The listing builds one solid part. Answer for the finished solid, in the listing's coordinates (mm). A direction names the side the tool comes from. Give positions to 0.01 mm unless a question says otherwise; leave off trailing zeros. Order: outer loops, then holes, each group sorted by start corner. A loop starts at its lowest first (then second) coordinate and runs counter-clockwise, first axis right, second up. Notation, with made-up numbers: (74, -13.5) -> (119, -13.5) arc R11 ccw to (119, -7.5) -> close; hole circle Ø8 at (87.5, 64.5). An arc over 180 degrees is marked (long way). Write item = value, one per line. Start each with the question number.
```python
from build123d import *

# Parameters (mm, degrees)
F1_DEPTH = 45
F0_R     = 1.2
F2_DEPTH = 1.5


with BuildPart() as f1:
    # F0 (on Top) → F1 (new body)
    with BuildSketch(Plane.XY):
        with BuildLine():
            Line((-13.376313, -16.508007), (-13.376313, -5.371486))
            ThreePointArc((-13.376313, -5.371486), (-27.376313, -1.436818), (-41.376313, -5.371486))
            Line((-41.376313, -5.371486), (-41.376313, -16.508007))
            ThreePointArc((-41.376313, -16.508007), (-27.376313, -20.442675), (-13.376313, -16.508007))
        make_face()
        with BuildLine():
            Line((-40.376313, -15.939747), (-40.376313, -5.939747))
            ThreePointArc((-40.376313, -5.939747), (-27.376313, -2.436818), (-14.376313, -5.939747))
            Line((-14.376313, -5.939747), (-14.376313, -15.939747))
            ThreePointArc((-14.376313, -15.939747), (-27.376313, -19.442675), (-40.376313, -15.939747))
        make_face(mode=Mode.SUBTRACT)
    extrude(amount=F1_DEPTH)

    # F0 (on Top) → F2 (join)
    with BuildSketch(Plane.XY):
        with BuildLine():
            ThreePointArc((-14.376313, -5.939747), (-27.376313, -2.436818), (-40.376313, -5.939747))
            Line((-40.376313, -5.939747), (-40.376313, -15.939747))
            ThreePointArc((-40.376313, -15.939747), (-27.376313, -19.442675), (-14.376313, -15.939747))
            Line((-14.376313, -15.939747), (-14.376313, -5.939747))
        make_face()
        with Locations((-32.828095, -16.290346)):
            Circle(F0_R, mode=Mode.SUBTRACT)
        with Locations((-28.928095, -16.290346)):
            Circle(F0_R, mode=Mode.SUBTRACT)
        with Locations((-36.702558, -12.947978)):
            Circle(F0_R, mode=Mode.SUBTRACT)
        with Locations((-32.828095, -12.947978)):
            Circle(F0_R, mode=Mode.SUBTRACT)
        with Locations((-28.928095, -12.947978)):
            Circle(F0_R, mode=Mode.SUBTRACT)
        with Locations((-25.028095, -16.290346)):
            Circle(F0_R, mode=Mode.SUBTRACT)
        with Locations((-21.128095, -16.290346)):
            Circle(F0_R, mode=Mode.SUBTRACT)
        with Locations((-25.028095, -12.947978)):
            Circle(F0_R, mode=Mode.SUBTRACT)
        with Locations((-21.128095, -12.947978)):
            Circle(F0_R, mode=Mode.SUBTRACT)
        with Locations((-17.228095, -12.947978)):
            Circle(F0_R, mode=Mode.SUBTRACT)
        with Locations((-36.702558, -9.047978)):
            Circle(F0_R, mode=Mode.SUBTRACT)
        with Locations((-32.828095, -9.047978)):
            Circle(F0_R, mode=Mode.SUBTRACT)
        with Locations((-28.928095, -9.047978)):
            Circle(F0_R, mode=Mode.SUBTRACT)
        with Locations((-32.828095, -5.190346)):
            Circle(F0_R, mode=Mode.SUBTRACT)
        with Locations((-28.928095, -5.190346)):
            Circle(F0_R, mode=Mode.SUBTRACT)
        with Locations((-25.028095, -9.047978)):
            Circle(F0_R, mode=Mode.SUBTRACT)
        with Locations((-21.128095, -9.047978)):
            Circle(F0_R, mode=Mode.SUBTRACT)
        with Locations((-17.228095, -9.047978)):
            Circle(F0_R, mode=Mode.SUBTRACT)
        with Locations((-25.028095, -5.190346)):
            Circle(F0_R, mode=Mode.SUBTRACT)
        with Locations((-21.128095, -5.190346)):
            Circle(F0_R, mode=Mode.SUBTRACT)
    extrude(amount=F2_DEPTH)


solid = f1.part
```
Item 1: A cutting plane is placed at B-B, the plane x = -32.25. Write down the section's boundary in (y, z).
Item 2: Consider L1, parallel to X at y = -13.75, z = 43; L2, parallel to Y at x = -28, z = 40; L3, parallel to Z at x = -37.5, y = -16.5. Determine where each line is inside the solid, lowest interval first. Write a range as from..to.
Item 3: A cutting plane is placed at C-C, the plane x = -36.5. Write down the section's boundary in (y, z), plus the area to 3 significant figures.
Item 4: The mould has two halves that part along X. Classify faces 3 (the flat face through (-41.376, -11, 22)), 4 (the cylindrical face through (-27.17, -1.438, 22.185)), 5 (the cylindrical face through (-16.084, -12.588, 0.74)): +X half, -X half, draft (parallel to the pull), parting line (faces both ways), or undercut.
Item 5: Which of the six approach directions +Z, -Z, +X, -X, +Y, -Y give full straight-line access (tool end or side, diameter ignored) to faces 1 (the cylindrical face through (-27.186, -19.442, 22.946)), 2 (the cylindrical face through (-22.327, -5.138, 0.74))?
Item 6: Flat-ended cylindrical pins translate along their axes: pin 1 (4 mm diameter, centred on x = -32.83, y = -12.95, fed in from +Z); pin 2 (4 mm diameter, centred on x = -31.5, z = 35.5, fed in from -Y); pin 3 (1.5 mm diameter, centred on x = -30.5, z = 10, fed in from -Y). Find the tip coordinate at first contact, or state that the pin passes through.
Item 7: A cutting plane is placed at A-A, the plane z = 19.5. Write down the section's boundary in (x, y), plus the area to 3 significant figures.
Item 8: A cutting plane is placed at D-D, the plane x = -28.5. Write down the section's boundary in (y, z), plus the area to 3 significant figures.
Check values:
q1.outline = (-20, 0) -> (-17.34, 0) -> (-17.34, 1.5) -> (-18.98, 1.5) -> (-18.98, 45) -> (-20, 45) -> close; (-15.24, 0) -> (-14, 0) -> (-14, 1.5) -> (-15.24, 1.5) -> close; (-11.9, 0) -> (-10.1, 0) -> (-10.1, 1.5) -> (-11.9, 1.5) -> close; (-8, 0) -> (-6.24, 0) -> (-6.24, 1.5) -> (-8, 1.5) -> close; (-4.14, 0) -> (-1.88, 0) -> (-1.88, 45) -> (-2.9, 45) -> (-2.9, 1.5) -> (-4.14, 1.5) -> close
q2.L1 = -41.38..-40.38, -14.38..-13.38
q2.L2 = -20.44..-19.44, -2.44..-1.44
q2.L3 = 0..1.5
q3.outline = (-18.85, 0) -> (-14.13, 0) -> (-14.13, 1.5) -> (-17.78, 1.5) -> (-17.78, 45) -> (-18.85, 45) -> close; (-11.77, 0) -> (-10.23, 0) -> (-10.23, 1.5) -> (-11.77, 1.5) -> close; (-7.87, 0) -> (-3.03, 0) -> (-3.03, 45) -> (-4.1, 45) -> (-4.1, 1.5) -> (-7.87, 1.5) -> close
q3.area = 109 mm^2
q4.face_3 = -X half
q4.face_4 = parting line
q4.face_5 = undercut
q5.face_1 = +Z
q5.face_2 = +Z, -Z
q6.pin_1 = 1.5
q6.pin_2 = -20.36
q6.pin_3 = -20.34
q7.outline = (-41.38, -16.51) arc R26.87 ccw to (-13.38, -16.51) -> (-13.38, -5.37) arc R26.87 ccw to (-41.38, -5.37) -> close; hole (-40.38, -15.94) arc R25.87 ccw to (-14.38, -15.94) -> (-14.38, -5.94) arc R25.87 ccw to (-40.38, -5.94) -> close
q7.area = 77.8 mm^2
q8.outline = (-20.42, 0) -> (-17.41, 0) -> (-17.41, 1.5) -> (-19.42, 1.5) -> (-19.42, 45) -> (-20.42, 45) -> close; (-15.17, 0) -> (-14.07, 0) -> (-14.07, 1.5) -> (-15.17, 1.5) -> close; (-11.83, 0) -> (-10.17, 0) -> (-10.17, 1.5) -> (-11.83, 1.5) -> close; (-7.93, 0) -> (-6.31, 0) -> (-6.31, 1.5) -> (-7.93, 1.5) -> close; (-4.07, 0) -> (-1.46, 0) -> (-1.46, 45) -> (-2.46, 45) -> (-2.46, 1.5) -> (-4.07, 1.5) -> close
q8.area = 102 mm^2
